```python
from build123d import *

# Parameters (mm, degrees)
SKETCH1_W           = 50
SKETCH1_H           = 36
SKETCH1_R           = 3.5
SKETCH1_R_2         = 1.7
BOSS_EXTRUDE1_DEPTH = 3.175
SKETCH2_R           = 4.5
CUT_EXTRUDE1_DEPTH  = 2


with BuildPart() as part:
    # Sketch1 → Boss-Extrude1 (new body)
    with BuildSketch(Plane(origin=(0, 0, 0), x_dir=(1, 0, 0), z_dir=(0, 1, 0))):
        with Locations((25, 18)):
            Rectangle(SKETCH1_W, SKETCH1_H)
        with Locations((13, 6.5)):
            Circle(SKETCH1_R, mode=Mode.SUBTRACT)
        with Locations((5, 5)):
            Circle(SKETCH1_R_2, mode=Mode.SUBTRACT)
        with Locations((5, 31)):
            Circle(SKETCH1_R_2, mode=Mode.SUBTRACT)
        with Locations((45, 31)):
            Circle(SKETCH1_R_2, mode=Mode.SUBTRACT)
        with Locations((45, 5)):
            Circle(SKETCH1_R_2, mode=Mode.SUBTRACT)
        with Locations((23, 6.5)):
            Circle(SKETCH1_R, mode=Mode.SUBTRACT)
        with Locations((33, 6.5)):
            Circle(SKETCH1_R, mode=Mode.SUBTRACT)
        with Locations((23, 16.5)):
            Circle(SKETCH1_R, mode=Mode.SUBTRACT)
        with Locations((33, 16.5)):
            Circle(SKETCH1_R, mode=Mode.SUBTRACT)
        with Locations((23, 26.5)):
            Circle(SKETCH1_R, mode=Mode.SUBTRACT)
        with Locations((33, 26.5)):
            Circle(SKETCH1_R, mode=Mode.SUBTRACT)
        with Locations((13, 16.5)):
            Circle(SKETCH1_R, mode=Mode.SUBTRACT)
        with Locations((13, 26.5)):
            Circle(SKETCH1_R, mode=Mode.SUBTRACT)
    extrude(amount=BOSS_EXTRUDE1_DEPTH)

    # Sketch2 → Cut-Extrude1 (cut)
    with BuildSketch(Plane(origin=(0, 3.175, 0), x_dir=(1, 0, 0), z_dir=(0, 1, 0))):
        with Locations((13, 26.5)):
            Circle(SKETCH2_R)
        with Locations((23, 26.5)):
            Circle(SKETCH2_R)
        with Locations((33, 26.5)):
            Circle(SKETCH2_R)
        with Locations((23, 16.5)):
            Circle(SKETCH2_R)
        with Locations((33, 16.5)):
            Circle(SKETCH2_R)
        with Locations((23, 6.5)):
            Circle(SKETCH2_R)
        with Locations((33, 6.5)):
            Circle(SKETCH2_R)
        with Locations((13, 16.5)):
            Circle(SKETCH2_R)
        with Locations((13, 6.5)):
            Circle(SKETCH2_R)
    extrude(amount=-CUT_EXTRUDE1_DEPTH, mode=Mode.SUBTRACT)


solid = part.part
```
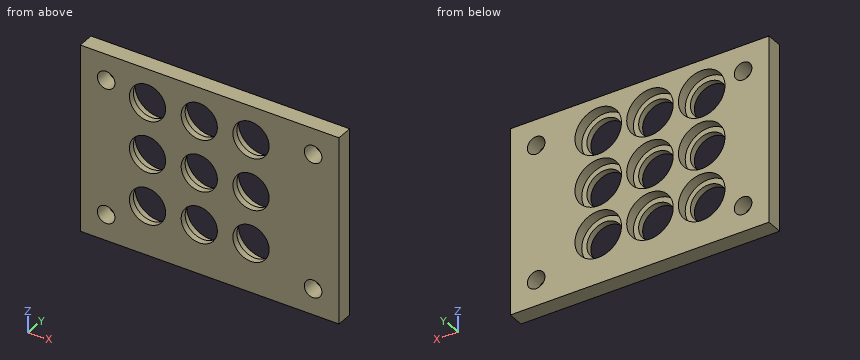
Work out the finished part from the listing and answer in its coordinate system (mm). Give positions to 0.01 mm unless a question says otherwise; leave off trailing zeros. Loops run counter-clockwise (first coordinate to the right, second up) from the corner with the lowest first, then second, coordinate; pieces in that order, holes last. Notation, with made-up numbers: (86, 36.25) -> (139, 36.25) arc R16 ccw to (139, 40.25) -> close; hole circle Ø5 at (-38, -33). An arc over 180 degrees is marked (long way). Use CSV: the item, a comma, the result in double quotes.
1. A flat-ended cylindrical pin translates along its axis: pin 1 Ø4.5 at (x, z) = (32.5, -28) entering from +Y (3 decimals). Find the tip coordinate at first contact, or state that the pin passes through.
Found:
pin 1,"y = 1.175"
2. The part is cut by section C-C (z = -26.5). Write down the section's boundary in (x, y) (3 decimals).
Found:
outline,"(0, 0) -> (9.5, 0) -> (9.5, 1.175) -> (8.5, 1.175) -> (8.5, 3.175) -> (0, 3.175) -> close; (16.5, 0) -> (19.5, 0) -> (19.5, 1.175) -> (18.5, 1.175) -> (18.5, 3.175) -> (17.5, 3.175) -> (17.5, 1.175) -> (16.5, 1.175) -> close; (26.5, 0) -> (29.5, 0) -> (29.5, 1.175) -> (28.5, 1.175) -> (28.5, 3.175) -> (27.5, 3.175) -> (27.5, 1.175) -> (26.5, 1.175) -> close; (36.5, 0) -> (50, 0) -> (50, 3.175) -> (37.5, 3.175) -> (37.5, 1.175) -> (36.5, 1.175) -> close"
3. The part is cut by section A-A (x = 45). Write down the section's boundary in (y, z) (3 decimals), then the cut area to 3 significant figures.
Found:
outline,"(0, -36) -> (3.175, -36) -> (3.175, -32.7) -> (0, -32.7) -> close; (0, -29.3) -> (3.175, -29.3) -> (3.175, -6.7) -> (0, -6.7) -> close; (0, -3.3) -> (3.175, -3.3) -> (3.175, 0) -> (0, 0) -> close"
area,"92.7 mm^2"
4. The part is cut by section B-B (y = 2.45). State how many separate pieces and enclosed holes the cut face has, then the cut area to 3 significant figures.
Found:
separate pieces,"1"
enclosed holes,"13"
area,"1,190 mm^2"
5. Straight lines are drawn through the part: line 1 (X direction, y = 1, z = -26.5); line 2 (Z direction, x = 13, y = 0.5); line 3 (X direction, y = 2.7, z = -26.5). For each, find the intervals that lie inside material, in ascending order.
Found:
line 1,"0 to 9.5, 16.5 to 19.5, 26.5 to 29.5, 36.5 to 50"
line 2,"-36 to -30, -23 to -20, -13 to -10, -3 to 0"
line 3,"0 to 8.5, 17.5 to 18.5, 27.5 to 28.5, 37.5 to 50"
6. The part is cut by section D-D (x = 21). Write down the section's boundary in (y, z) (3 decimals), then the cut area to 3 significant figures.
Found:
outline,"(0, -36) -> (3.175, -36) -> (3.175, -30.531) -> (1.175, -30.531) -> (1.175, -29.372) -> (0, -29.372) -> close; (0, -23.628) -> (1.175, -23.628) -> (1.175, -22.469) -> (3.175, -22.469) -> (3.175, -20.531) -> (1.175, -20.531) -> (1.175, -19.372) -> (0, -19.372) -> close; (0, -13.628) -> (1.175, -13.628) -> (1.175, -12.469) -> (3.175, -12.469) -> (3.175, -10.531) -> (1.175, -10.531) -> (1.175, -9.372) -> (0, -9.372) -> close; (0, -3.628) -> (1.175, -3.628) -> (1.175, -2.469) -> (3.175, -2.469) -> (3.175, 0) -> (0, 0) -> close"
area,"45.7 mm^2"
